Part model, mm, in its own coordinate system. Face numbers are marked on the shaded views. A direction names the side the tool comes from. Round coordinates to 2 decimals unless told otherwise and drop trailing zeros. Order: outer loops, then holes, each group sorted by start corner. A loop starts at its lowest first (then second) coordinate and runs counter-clockwise, first axis right, second up. Notation, with made-up numbers: M -35,77.5 L -12,77.5 A29 cw -12,97.5 Z; hole C 36,52 d6. An arc over 180 degrees is marked long. Write each question's results on one line, items separated by ' | '. Start each with the question number.
1. Which spindle directions (+Z, -Z, +X, -X, +Y, -Y) get a long thin tool onto all of the face, cutting with end or side? Do the marked faces 1 and 2. Say none if no direction does.
2. Band-saw the part on A-A, the plane y = 0.5. List the corners of the cut face in (x, z), then the cut area to 3 significant figures.
3. Band-saw the part on D-D, the plane y = 2.25. List the corners of the cut face in (x, z).
4. Band-saw the part on B-B, the plane z = 1.5. List the corners of the cut face in (x, y) (3 decimals), then the cut area to 3 significant figures.
5. Band-saw the part on C-C, the plane x = 0. List the corners of the cut face in (y, z) (3 decimals), then the cut area to 4 significant figures.
6. Drop flat-ended pins along their axis: pin 1 Ø2 at (x, y) = (-2, -1) entering from +Z; pin 2 Ø1.1 at (y, z) = (0.5, 2) entering from -X. Give the stop position or say it passes through.
7. Probe L1, parallel to X at y = -1.25, z = 2.25; L2, parallel to X at y = 0.5, z = 1.5; L3, parallel to X at y = -0.25, z = 1.25. List the from-to ranges inside material, lowest first. Write a range as [from, to].
8. Two-plate mould, pull along X, no slides. Class the marked faces 3, 4 and 5: +X half, -X half, draft (parallel to the pull), parting line (faces both ways), or undercut.
```python
from build123d import *

# Parameters (mm, degrees)
BASE_FLANGE1_DEPTH  = 2.5
SKETCH3_W           = 0.4
SKETCH3_H           = 3.67
BOSS_EXTRUDE1_DEPTH = 4.5
SKETCH5_W           = 3.4
SKETCH5_H           = 1
CUT_EXTRUDE1_DEPTH  = 4.5
FILLET1_RADIUS      = 1.335
FILLET1_LENGTH      = 0.4


# Sheet-metal steps are written as plain solids
with BuildPart() as part:
    # Sketch2 → Base-Flange1 (new body)
    with BuildSketch(Plane.XY):
        with BuildLine():
            Line((0.71, -1.835), (0.71, 1.835))
            ThreePointArc((0.71, 1.835), (0, 2.545), (-0.71, 1.835))
            Line((-0.71, 1.835), (-0.71, -2.335))
            ThreePointArc((-0.71, -2.335), (-1.268334084, -3.292391266), (-2.376541882, -3.277884031))
            Line((-2.376541882, -3.277884031), (-7.090962036, -0.445174619))
            Line((-7.090962036, -0.445174619), (-6.884946806, -0.102307698))
            Line((-6.884946806, -0.102307698), (-2.170526652, -2.93501711))
            ThreePointArc((-2.170526652, -2.93501711), (-1.465303508, -2.944248987), (-1.11, -2.335))
            Line((-1.11, -2.335), (-1.11, 1.835))
            ThreePointArc((-1.11, 1.835), (0, 2.945), (1.11, 1.835))
            Line((1.11, 1.835), (1.11, -1.835))
            Line((1.11, -1.835), (0.71, -1.835))
        make_face()
    extrude(amount=BASE_FLANGE1_DEPTH)

    # Sketch3 → Boss-Extrude1 (add)
    with BuildSketch(Plane.XY.offset(2.5)):
        with Locations((0.91, 0)):
            Rectangle(SKETCH3_W, SKETCH3_H)
    extrude(amount=BOSS_EXTRUDE1_DEPTH)

    # Sketch5 → Cut-Extrude1 (cut)
    with BuildSketch(Plane(origin=(1.11, 0, 0), x_dir=(0, 0, -1), z_dir=(1, 0, 0))):
        with Locations((-5.3, -1.335)):
            Rectangle(SKETCH5_W, SKETCH5_H)
    extrude(amount=-CUT_EXTRUDE1_DEPTH, mode=Mode.SUBTRACT)

    # Fillet1: full round fillet: the end face becomes a half cylinder, R = half its width
    fillet1_face = Plane((0.91, 0.5, 7), x_dir=(-1, 0, 0), z_dir=(0, 0, 1))  # on the end face: x along it, z out of the body
    fillet1_slab = fillet1_face.offset(-FILLET1_RADIUS / 2) * Box(FILLET1_LENGTH, 2 * FILLET1_RADIUS, FILLET1_RADIUS, mode=Mode.PRIVATE)  # the body's end, R deep
    fillet1_round = Plane((0.91, 0.5, 5.665), x_dir=(0, 0, 1), z_dir=(-1, 0, 0)) * Cylinder(FILLET1_RADIUS, FILLET1_LENGTH, mode=Mode.PRIVATE)  # its axis R under the face
    add(fillet1_slab - fillet1_round, mode=Mode.SUBTRACT)


solid = part.part
```
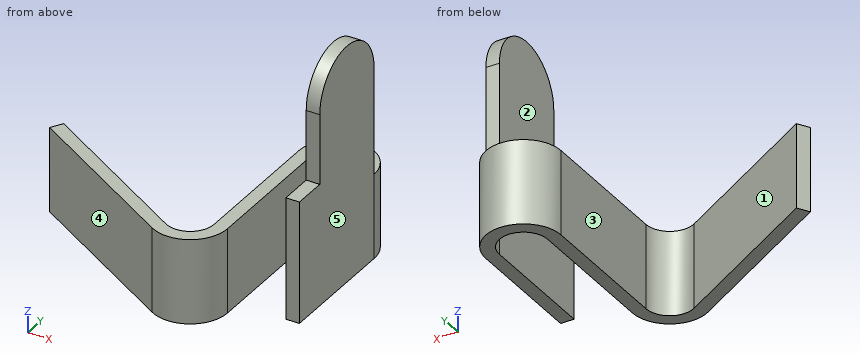
Solution:
1) face 1: +Z, -Z, +Y | face 2: +Z, -Z, -Y
2) outline: M -1.11,0 L -0.71,0 L -0.71,2.5 L -1.11,2.5 Z; M 0.71,0 L 1.11,0 L 1.11,7 L 0.71,7 Z | area: 3.80 mm^2
3) outline: M -1.03,0 L -0.58,0 L -0.58,2.5 L -1.03,2.5 Z; M 0.58,0 L 1.03,0 L 1.03,2.5 L 0.58,2.5 Z
4) outline: M -7.091,-0.445 L -2.377,-3.278 A1.1 ccw -0.71,-2.335 L -0.71,1.835 A0.71 cw 0.71,1.835 L 0.71,-1.835 L 1.11,-1.835 L 1.11,1.835 A1.11 ccw -1.11,1.835 L -1.11,-2.335 A0.7 cw -2.171,-2.935 L -6.885,-0.102 Z | area: 7.24 mm^2
5) outline: M 2.545,0 L 2.945,0 L 2.945,2.5 L 2.545,2.5 Z | area: 1.000 mm^2
6) pin 1: z = 2.5 | pin 2: x = -1.11
7) L1: [-5.75, -4.97], [-1.11, -0.71], [0.71, 1.11] | L2: [-1.11, -0.71], [0.71, 1.11] | L3: [-6.97, -6.64], [-1.11, -0.71], [0.71, 1.11]
8) face 3: undercut | face 4: -X half | face 5: +X half
